Source: CAD feature listing. Evaluate the final solid. Frame: model axes, mm. A direction names the side the tool comes from. Round coordinates to 2 decimals unless told otherwise and drop trailing zeros. Order: outer loops, then holes, each group sorted by start corner. A loop starts at its lowest first (then second) coordinate and runs counter-clockwise, first axis right, second up. Notation, with made-up numbers: (34.25, 34) - (48.25, 34) arc R20 ccw to (48.25, 46) - close; hole circle Ø11 at (-8.5, 81.25). An arc over 180 degrees is marked (long way). Put each result on its own line as item: value. Start each with the question number.
1) Section A-A on z = 7.25. Output: boundary loops of the cut face in (x, y).
2) Section B-B on y = 5. Output: boundary loops of the cut face in (x, z).
3) Access query for faces 1 (the face through (6, 11.3, 6)), 2 (the face through (16.4, 9, 6)). Directions: +Z, -Z, +X, -X, +Y, -Y. A direction counts if a zero-diameter tool reaches every point of the face in a straight line with its end or side. Return the directions, or none.
4) Section C-C on x = 9.25. Output: boundary loops of the cut face in (y, z), then the cut area to 3 significant figures.
5) Section D-D on z = 10.5. Output: boundary loops of the cut face in (x, y).
6) Line query: probe 1 along Y at (x, z) = (1, 6.75); probe 2 along X at (y, z) = (11, 9.25); probe 3 along X at (y, z) = (13, 10.5). Output: solid intervals per line, ascending. Write a range as [from, to].
7) Contact query for flat-ended pins moving along their axis: P1, Ø5.5, axis at y = 5, z = 6, coming from the -X side; P2, Ø5.5, axis at x = 5, z = 4, coming from the -Y side. Output: stop coordinate, or through.
```python
from build123d import *

# Parameters (mm, degrees)
F0_W     = 16.4
F0_H     = 19.2
F1_DEPTH = 11.3
F2_W     = 11.3
F2_H     = 11.3
F3_DEPTH = 25
F4_R     = 2
F5_R     = 1


with BuildPart() as f1:
    # F0 (on Top) → F1 (new body)
    with BuildSketch(Plane.XY):
        with Locations((8.2, 9.6)):
            Rectangle(F0_W, F0_H)
    extrude(amount=F1_DEPTH)

    # F2 (on face) → F3 (cut)
    with BuildSketch(Plane.XY.offset(11.3)):
        with Locations((5.65, 5.65)):
            Rectangle(F2_W, F2_H)
    extrude(amount=-F3_DEPTH, mode=Mode.SUBTRACT)

    # F4
    f4_edges = [f1.edges().sort_by_distance(p)[0] for p in [
        (13.85, 0, 0),
        (0, 15.25, 0),
        (13.85, 0, 11.3),
        (0, 15.25, 11.3),
    ]]
    fillet(f4_edges, radius=F4_R)

    # F5
    f5_edges = [f1.edges().sort_by_distance(p)[0] for p in [
        (16.4, 19.2, 5.65),
    ]]
    fillet(f5_edges, radius=F5_R)


solid = f1.part
```
Answer sheet:
1. outline: (0, 11.3) - (11.3, 11.3) - (11.3, 0) - (16.4, 0) - (16.4, 18.2) arc R1 ccw to (15.4, 19.2) - (0, 19.2) - close
2. outline: (11.3, 0) - (16.4, 0) - (16.4, 11.3) - (11.3, 11.3) - close
3. face 1: +Z, -Z, -X, -Y
3. face 2: +Z, -Z, +X, +Y, -Y
4. outline: (11.3, 0) - (19.2, 0) - (19.2, 11.3) - (11.3, 11.3) - close
4. area: 89.3 mm^2
5. outline: (0.4, 11.3) - (11.3, 11.3) - (11.3, 0.4) - (16.4, 0.4) - (16.4, 18.2) arc R1 ccw to (15.4, 19.2) - (0.4, 19.2) - close
6. probe 1: [11.3, 19.2]
6. probe 2: [11.3, 16.4]
6. probe 3: [0.4, 16.4]
7. P1: x = 11.3
7. P2: y = 11.3
